Can you work these out from the drawing? Everything is in mm from the part's minimum corner. Round coordinates to 2 decimals unless told otherwise and drop trailing zeros. Write each loop counter-clockwise with the first axis right and the second up, starting at its lowest first coordinate (ties: lowest second). Pieces come first, ordered by that corner, then holes. Notation, with made-up numbers: (60.25, 47) -> (102.25, 47) arc R36 cw to (102.25, 81) -> close; hole circle Ø4 at (72, 65.25). An arc over 180 degrees is marked (long way). Write item = value, one per line. Start each with the question number.
1) Imagine slicing it at C-C, the plane z = 91. Please give me the cut outline in (x, y).
2) Imagine slicing it at D-D, the plane x = 1083. Please give me the cut outline in (y, z).
3) If I drill on line 1 (X direction, y = 1304, z = 793.5); line 2 (Y direction, x = 1169.5, z = 106), over which ranges is the centre line in solid material (lowest first)?
4) Imagine slicing it at B-B, the plane z = 431. Please give me the cut outline in (x, y).
5) Imagine slicing it at A-A, the plane y = 1352.5. Please give me the cut outline in (x, z), then the cut area to 3 significant figures.
6) Thinking about a two-plate mould opening in X: for the marked faces 1, 2 and 3, which applies, +X half, -X half, draft (parallel to the pull), parting line (faces both ways), or undercut?
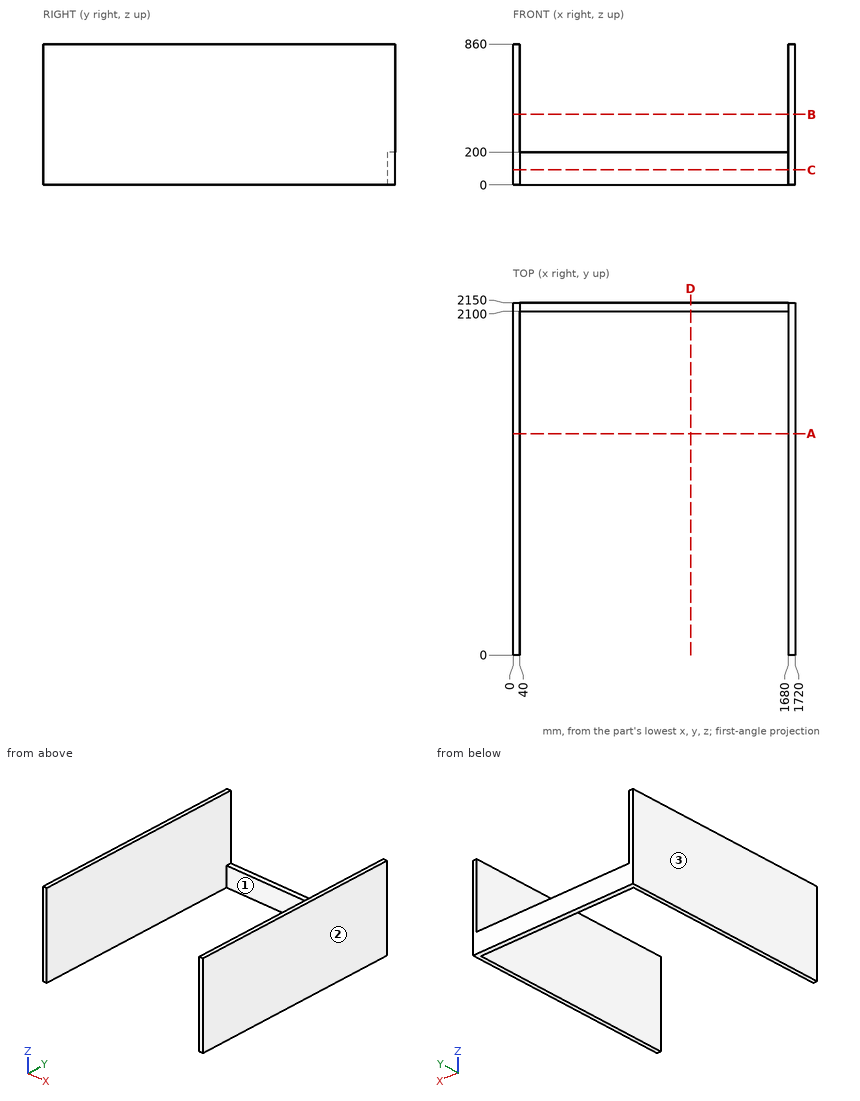
Reported:
q1.outline = (0, 0) -> (40, 0) -> (40, 2100) -> (1680, 2100) -> (1680, 0) -> (1720, 0) -> (1720, 2150) -> (0, 2150) -> close
q2.outline = (2100, 0) -> (2150, 0) -> (2150, 200) -> (2100, 200) -> close
q3.line_1 = 0 to 40, 1680 to 1720
q3.line_2 = 2100 to 2150
q4.outline = (0, 0) -> (40, 0) -> (40, 2150) -> (0, 2150) -> close; (1680, 0) -> (1720, 0) -> (1720, 2150) -> (1680, 2150) -> close
q5.outline = (0, 0) -> (40, 0) -> (40, 860) -> (0, 860) -> close; (1680, 0) -> (1720, 0) -> (1720, 860) -> (1680, 860) -> close
q5.area = 68,800 mm²
q6.face_1 = undercut
q6.face_2 = +X half
q6.face_3 = -X half
